The drawing under review shows one solid part. Ordinate dimensions are in mm from its lowest x, y, z. A direction names the side the tool comes from. Round coordinates to 2 decimals unless told otherwise and drop trailing zeros. Write each loop counter-clockwise with the first axis right and the second up, starting at its lowest first coordinate (ties: lowest second). Pieces come first, ordered by that corner, then holes. Notation, with made-up numbers: (52, 27.25) -> (100, 27.25) arc R27 cw to (100, 54.25) -> close; hole circle Ø1 at (65, 63). An arc over 180 degrees is marked (long way). Use CSV: the item, a comma, the result in double quotes. Start each with the question number.
1) Machinability: for the marked faces 1 and 2, which of the approach directions +Z, -Z, +X, -X, +Y, -Y give a long, thin tool a straight path to every point of the face, cutting with its end or side? Answer none if there is none.
2) Wall thickness on probe 1 along X at (y, z) = (9.5, 11); probe 2 along Z at (x, y) = (2, 21); probe 3 along Z at (x, y) = (1.5, 25): over which ranges is each line inside the solid? List them lowest first. Write a range as [from, to].
3) Take a section at C-C, the plane z = 25.5. Give the boundary of the cut face in (x, y).
4) Take a section at A-A, the plane x = 12. Give the boundary of the cut face in (y, z).
5) Take a section at D-D, the plane x = 3.75. Give the boundary of the cut face in (y, z).
6) Mouldability with a two-part tool opening along Z and no side actions: class the marked faces 3, 4, 5 and 6 as released by +Z, released by -Z, zero draft, split by the parting line, or undercut.
7) For pin 1 Ø2 at (y, z) = (7, 27) entering from -X, flat-tipped, find the tip position at first contact; note if it passes through.
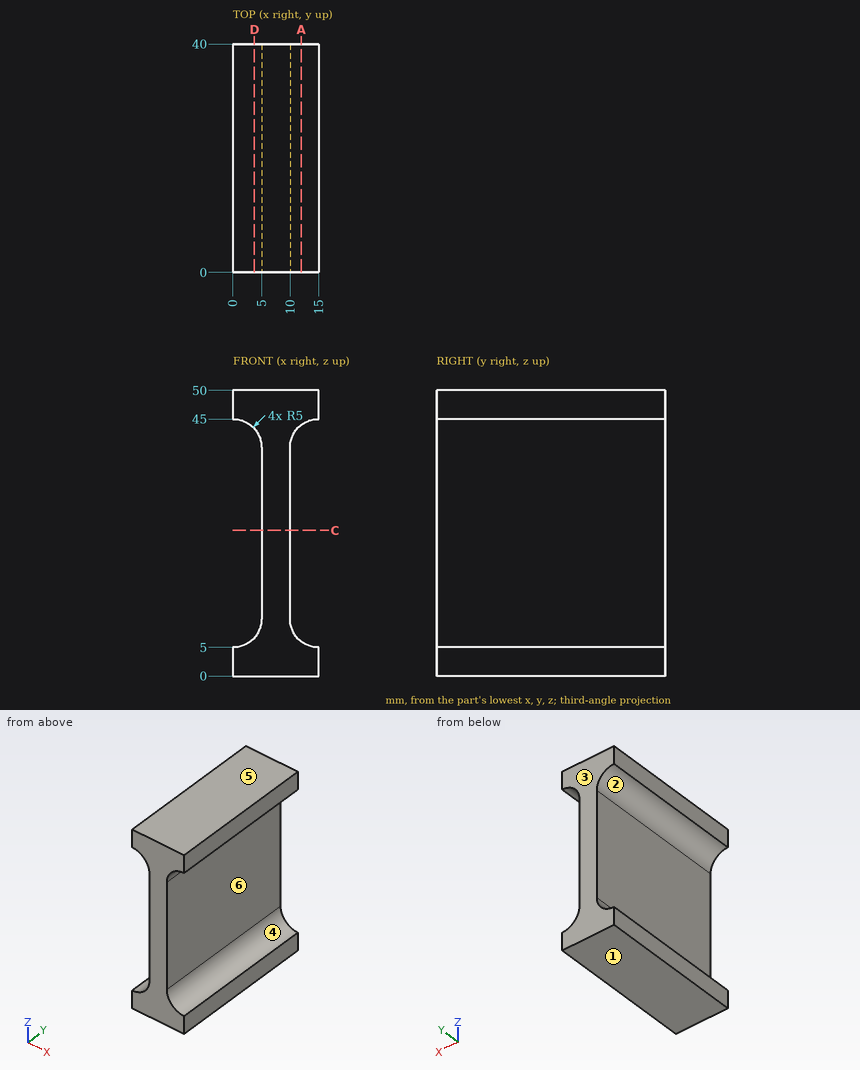
Values found:
1,face 1,"-Z, +X, -X, +Y, -Y"
1,face 2,"-X, +Y, -Y"
2,probe 1,"[5, 10]"
2,probe 2,"[0, 5.42], [44.58, 50]"
2,probe 3,"[0, 5.23], [44.77, 50]"
3,outline,"(5, 0) -> (10, 0) -> (10, 40) -> (5, 40) -> close"
4,outline,"(0, 0) -> (40, 0) -> (40, 6) -> (0, 6) -> close; (0, 44) -> (40, 44) -> (40, 50) -> (0, 50) -> close"
5,outline,"(0, 0) -> (40, 0) -> (40, 6.69) -> (0, 6.69) -> close; (0, 43.31) -> (40, 43.31) -> (40, 50) -> (0, 50) -> close"
6,face 3,"zero draft"
6,face 4,"undercut"
6,face 5,"released by +Z"
6,face 6,"undercut"
7,pin 1,"x = 5"
